from build123d import *

# Parameters (mm, degrees)
F0_R     = 5
F1_DEPTH = 10


with BuildPart() as f1:
    # F0 (on Front) → F1 (new body)
    with BuildSketch(Plane.XZ):
        Polygon((-10, 20), (-40, 20), (-40, 10), (-25, 10), (-25, -10), (-40, -10), (-40, -20), (-10, -20), (-10, -15), (10, -15), (10, -20), (40, -20), (40, -10), (25, -10), (25, 10), (40, 10), (40, 20), (10, 20), (10, 15), (-10, 15), align=None)
        Circle(F0_R, mode=Mode.SUBTRACT)
    extrude(amount=F1_DEPTH)


solid = f1.part
Here's how the part is built. I have some questions about the finished solid (model axes, mm). A direction names the side the tool comes from. Give positions to 0.01 mm unless a question says otherwise; leave off trailing zeros. Order: outer loops, then holes, each group sorted by start corner. A loop starts at its lowest first (then second) coordinate and runs counter-clockwise, first axis right, second up. Notation, with made-up numbers: (39.5, -36.75) -> (51.5, -36.75) arc R15 cw to (51.5, -10.75) -> close; hole circle Ø2 at (32.5, 72.5). An arc over 180 degrees is marked (long way). Use a Markdown table: item, result. Add a question column.
Item 1: For faces 5 (the face through (-32, -5, -10)), 6 (the face through (40, -5, 15)), 7 (the face through (32, -5, 10)), 8 (the face through (0, -5, 15)), 9 (the face through (-10, -5, -18)), which set-ups out of +Z, -Z, +X, -X, +Y, -Y let a thin tool reach every point of the face, with its end or its side?
Item 2: Imagine slicing it at A-A on z = 0. Please give me the cut outline in (x, y).
Item 3: Imagine slicing it at C-C on y = -4.25. Please give me the cut outline in (x, z), plus the area to 3 significant figures.
Item 4: Imagine slicing it at D-D on z = -6. Please give me the cut outline in (x, y), plus the area to 3 significant figures.
Item 5: Imagine slicing it at B-B on x = 3. Please give me the cut outline in (y, z).
Item 6: Will these pins go through, and if not, where does the flat tip stop? pin 1 (5 mm diameter, centred on y = -3, z = -0.5, fed in from +X); pin 2 (6 mm diameter, centred on x = 0, z = 0, fed in from -Y); pin 3 (6 mm diameter, centred on y = -8, z = 4.5, fed in from -X); pin 4 (5 mm diameter, centred on x = 0.5, y = -5, fed in from -Z).
Item 7: If we mould it in two halves opening along X, with no side actions, what happens to faces 1 (the face through (-40, -5, 15)), 2 (the face through (25, -5, 20)), 3 (the face through (0, -5, -15)), 4 (the face through (25, -5, 0))? For each: pulls with the +X half, pulls with the -X half, needs draft (parallel to the pull), parting line crosses it, or undercut.
Item 8: I need wall thicknesses on line 1 (Z direction, x = -33.5, y = -6); line 2 (Z direction, x = 0, y = -4.5); line 3 (X direction, y = -4.25, z = 18.5). Which ranges of each line are inside material? Lowest first, please.
Data:
| question | item | result |
|---|---|---|
| 1 | face 5 | -X, +Y, -Y |
| 1 | face 6 | +Z, -Z, +X, +Y, -Y |
| 1 | face 7 | +X, +Y, -Y |
| 1 | face 8 | +Z, +Y, -Y |
| 1 | face 9 | -Z, +Y, -Y |
| 2 | outline | (-25, -10) -> (-5, -10) -> (-5, 0) -> (-25, 0) -> close; (5, -10) -> (25, -10) -> (25, 0) -> (5, 0) -> close |
| 3 | outline | (-40, -20) -> (-10, -20) -> (-10, -15) -> (10, -15) -> (10, -20) -> (40, -20) -> (40, -10) -> (25, -10) -> (25, 10) -> (40, 10) -> (40, 20) -> (10, 20) -> (10, 15) -> (-10, 15) -> (-10, 20) -> (-40, 20) -> (-40, 10) -> (-25, 10) -> (-25, -10) -> (-40, -10) -> close; hole circle Ø10 at (0, 0) |
| 3 | area | 2,320 mm² |
| 4 | outline | (-25, -10) -> (25, -10) -> (25, 0) -> (-25, 0) -> close |
| 4 | area | 500 mm² |
| 5 | outline | (-10, -15) -> (0, -15) -> (0, -4) -> (-10, -4) -> close; (-10, 4) -> (0, 4) -> (0, 15) -> (-10, 15) -> close |
| 6 | pin 1 | stops at x = 25 |
| 6 | pin 2 | passes through |
| 6 | pin 3 | stops at x = -25 |
| 6 | pin 4 | stops at z = -15 |
| 7 | face 1 | pulls with the -X half |
| 7 | face 2 | needs draft |
| 7 | face 3 | undercut |
| 7 | face 4 | pulls with the +X half |
| 8 | line 1 | z = -20 to -10, 10 to 20 |
| 8 | line 2 | z = -15 to -5, 5 to 15 |
| 8 | line 3 | x = -40 to -10, 10 to 40 |
